Work out the finished part from the listing and answer in its coordinate system (mm). Face numbers are marked on the shaded views. A direction names the side the tool comes from. Round coordinates to 2 decimals unless told otherwise and drop trailing zeros. Order: outer loops, then holes, each group sorted by start corner. A loop starts at its lowest first (then second) coordinate and runs counter-clockwise, first axis right, second up.
Autodesk Inventor part; units mm, degrees
sketch "Эскиз1" plane through (0, 0, 0) normal (1, 0, 0) x (0, 1, 0)
  line L0 (25.8579, -14.1421) -> (-14.1421, -14.1421)
  line L1 (-14.1421, -14.1421) -> (-14.1421, 25.8579)
  arc A0 (25.8579, -14.1421) -> (-14.1421, 25.8579) centre (-14.1421, -14.1421) ccw
  line L2 (-14.1421, -14.1421) -> (14.1421, 14.1421) construction
  point P0 (0, 0)
  point P1 (0, 0)
  dimension "d0" = 40
extrude "Выдавливание1" add sketch "Эскиз1" along normal mid plane 210
sketch "Эскиз2" plane through (105, 25.8579, -14.1421) normal (0, 0, -1) x (-1, 0, 0)
  line L0 (210, 0) -> (0, 0)
  line L1 (0, -40) -> (0, 0)
  line L2 (210, -40) -> (0, -40)
  line L3 (210, 0) -> (210, -40)
  point P0 (105, -25.8579)
extrude "Выдавливание2" add sketch "Эскиз2" along normal blind 30
sketch "Эскиз3" plane through (-105, 25.8579, -14.1421) normal (0, 1, 0) x (1, 0, 0)
  line L0 (0, 0) -> (210, 0)
  line L1 (210, 0) -> (210, 30)
  line L2 (0, 30) -> (210, 30)
  line L3 (0, 0) -> (0, 30)
  point P0 (105, -14.1421)
extrude "Выдавливание3" cut sketch "Эскиз3" against normal blind 4
sketch "Эскиз5" plane through (-105, 21.8579, -14.1421) normal (0, 1, 0) x (1, 0, 0)
  line L0 (210, -40) -> (210, 30)
  line L1 (210, 15) -> (0, 15) construction
  line L2 (0, -40) -> (0, 30)
  line L3 (0, 30) -> (210, 30)
  circle A0 centre (45, 15) radius 2.55
  line L4 (270, 15) -> (60, 15) construction
  circle A1 centre (105, 15) radius 2.55
  line L5 (330, 15) -> (120, 15) construction
  circle A2 centre (165, 15) radius 2.55
  dimension "d7" = 15
  dimension "d8" = 5.1
  dimension "d9" = 45
  dimension "d12" = 60
extrude "Выдавливание4" cut sketch "Эскиз5" against normal up to next
sketch "Эскиз6" plane through (-105, 21.8579, 25.8579) normal (0, -1, 0) x (1, 0, 0)
  line L0 (-10, -65) -> (0, -60)
  line L1 (-10, -45) -> (-10, -65)
  line L2 (0, -50) -> (-10, -45)
  line L3 (0, -40) -> (0, -70)
  point P0 (105, -25.8579)
extrude "Выдавливание5" add sketch "Эскиз6" along normal blind 20
mirror "Зеркальное отражение1" about plane through (0, 0, 0) normal (1, 0, 0) of "Выдавливание5"
properties part number "Край_новой_крышки"
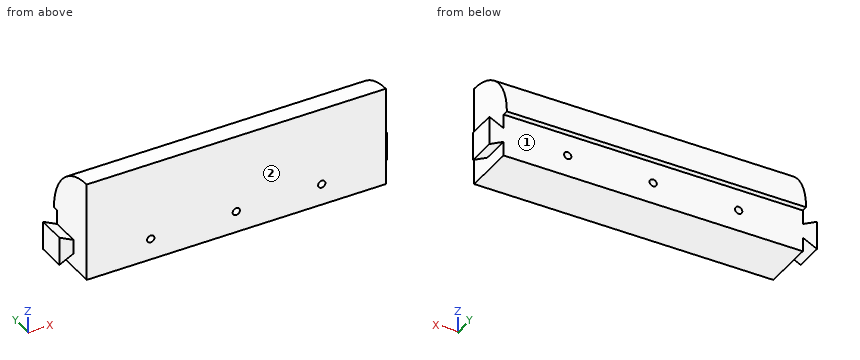
Item 1: Find section D-D (y = -6). Write down the section's boundary in (x, z).
Item 2: Find the intervals of material crossed by line 1 along X through (y, z) = (6.5, -21); line 2 along X through (y, z) = (2, -36); line 3 along Z through (x, y) = (0, -3), in increasing order.
Item 3: Find section B-B (y = 6). Write down the section's boundary in (x, z), plus the area to 3 significant figures.
Item 4: A tool of negligible diameter and unlimited length cuts with its end or side. For the marked faces 1 and 2, from which of +Z, -Z, +X, -X, +Y, -Y can it reach the whole face along a straight path? Write none if from no direction.
Item 5: Find section A-A (x = -60). Write down the section's boundary in (y, z).
Item 6: Given pin 1 (3 mm diameter, centred on y = 13, z = 6, fed in from -X); pin 2 (9 mm diameter, centred on x = 5.5, z = -30, fed in from +Y); pin 3 (6 mm diameter, centred on x = 53.5, y = -3.5, fed in from +Z), each flat-ended and moving along its own axis, determine where each tip first touches the part or whether it passes through.
Item 7: Find section C-C (z = 5.5). Write down the section's boundary in (x, y), plus the area to 3 significant figures.
Model answer:
1. outline: (-105, -44.14) - (105, -44.14) - (105, 25.02) - (-105, 25.02) - close; hole circle Ø5.1 at (-60, -29.14); hole circle Ø5.1 at (0, -29.14); hole circle Ø5.1 at (60, -29.14)
2. line 1: x = -115 to -111.28, -105 to 105, 111.28 to 115
2. line 2: x = -115 to -108.72, -105 to 105, 108.72 to 115
2. line 3: z = -44.14 to -31.69, -26.59 to 24.27
3. outline: (-115, -39.14) - (-105, -34.14) - (-105, -44.14) - (105, -44.14) - (105, -34.14) - (115, -39.14) - (115, -19.14) - (105, -24.14) - (105, 20.42) - (-105, 20.42) - (-105, -24.14) - (-115, -19.14) - close; hole circle Ø5.1 at (-60, -29.14); hole circle Ø5.1 at (0, -29.14); hole circle Ø5.1 at (60, -29.14)
3. area: 13,800 mm2
4. face 1: -Z, +X, -X, +Y
4. face 2: +Z, -Z, +X, -X, -Y
5. outline: (-14.14, -44.14) - (21.86, -44.14) - (21.86, -31.69) - (-14.14, -31.69) - close; (-14.14, -26.59) - (21.86, -26.59) - (21.86, -14.14) - (25.86, -14.14) arc R40 ccw to (-14.14, 25.86) - close
6. pin 1: stops at x = -105
6. pin 2: stops at y = 21.86
6. pin 3: stops at z = 25.12
7. outline: (-105, -14.14) - (105, -14.14) - (105, 20.7) - (-105, 20.7) - close
7. area: 7,320 mm2
